Here's how the part is built. I have some questions about the finished solid (model axes, mm). Face numbers are marked on the shaded views. A direction names the side the tool comes from. Coordinates: 2 decimals unless noted, no trailing zeros. Write each loop counter-clockwise with the first axis right and the second up, starting at its lowest first coordinate (ties: lowest second). Pieces come first, ordered by that corner, then holes.
```python
from build123d import *

# Parameters (mm, degrees)
SKETCH1_W                               = 125
SKETCH1_H                               = 40
BOSS_EXTRUDE1_DEPTH                     = 10
BOSS_EXTRUDE2_DEPTH                     = 10
SKETCH9_W                               = 58.70504164
SKETCH9_H                               = 3.000259145
CUT_EXTRUDE1_DEPTH                      = 67
FILLET1_R                               = 3
FILLET2_R                               = 3
CBORE_FOR_M8_HEX_HEAD_BOLT1_D           = 9
CBORE_FOR_M8_HEX_HEAD_BOLT1_CBORE_D     = 18.01
CBORE_FOR_M8_HEX_HEAD_BOLT1_CBORE_DEPTH = 5.68


with BuildPart() as part:
    # Sketch1 → Boss-Extrude1 (new body)
    with BuildSketch(Plane(origin=(0, 0, 0), x_dir=(1, 0, 0), z_dir=(0, 1, 0))):
        with Locations((62.5, 20)):
            Rectangle(SKETCH1_W, SKETCH1_H)
    extrude(amount=BOSS_EXTRUDE1_DEPTH)

    # Sketch4 → Boss-Extrude2 (add)
    with BuildSketch(Plane.XY):
        with BuildLine():
            Line((30.012948081, 0), (69.987051919, 0))
            Line((69.987051919, 0), (69.987051919, 35))
            ThreePointArc((69.987051919, 35), (50, 54.987051919), (30.012948081, 35))
            Line((30.012948081, 35), (30.012948081, 0))
        make_face()
    extrude(amount=-BOSS_EXTRUDE2_DEPTH)

    # Sketch9 → Cut-Extrude1 (cut)
    with BuildSketch(Plane.XY):
        with Locations((53.635144719, 1.500129573)):
            Rectangle(SKETCH9_W, SKETCH9_H)
    extrude(amount=-CUT_EXTRUDE1_DEPTH, mode=Mode.SUBTRACT)

    # Fillet1
    fillet1_edges = [part.edges().sort_by_distance(p)[0] for p in [
        (0, 5, 0),
        (125, 5, 0),
        (125, 5, -40),
        (0, 5, -40),
    ]]
    fillet(fillet1_edges, radius=FILLET1_R)

    # Fillet2
    fillet2_edges = [part.edges().sort_by_distance(p)[0] for p in [
        (82.987665539, 0, -20),
        (24.282623899, 0, -20),
    ]]
    fillet(fillet2_edges, radius=FILLET2_R)

    # CBORE for M8 Hex Head Bolt1 (through all)
    with Locations(Plane(origin=(50, 35, -10), x_dir=(-1, 0, 0), z_dir=(0, 0, -1))):
        with Locations((0, 0)):
            CounterBoreHole(CBORE_FOR_M8_HEX_HEAD_BOLT1_D / 2, CBORE_FOR_M8_HEX_HEAD_BOLT1_CBORE_D / 2, CBORE_FOR_M8_HEX_HEAD_BOLT1_CBORE_DEPTH)


solid = part.part
```
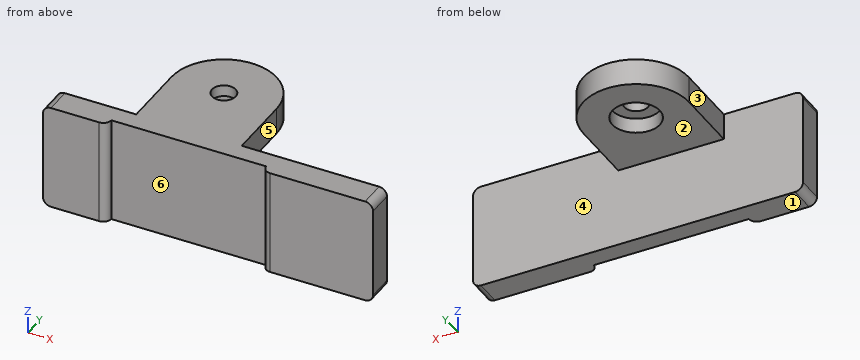
1) I need wall thicknesses on probe 1 along Y at (x, z) = (50, -6) (3 decimals); probe 2 along Y at (x, z) = (50, -1.75); probe 3 along Z at (x, y) = (51, 27). Which ranges of each line are inside material? Lowest first, please.
Values follow:
probe 1: y = 3 to 25.995, 44.005 to 54.987
probe 2: y = 3 to 30.5, 39.5 to 54.99
probe 3: z = -4.32 to 0
2) We'd pull the mould along X, two halves only. Please class the marked faces 4, 5 and 6: pulls with the +X half, pulls with the -X half, needs draft (parallel to the pull), parting line crosses it, or undercut.
Values follow:
face 4: needs draft
face 5: pulls with the +X half
face 6: undercut
3) Imagine slicing it at C-C on y = 23.5. Please give me the cut outline in (x, z), then the cut area to 3 significant figures.
Values follow:
outline: (30.01, -10) - (69.99, -10) - (69.99, 0) - (30.01, 0) - close
area: 400 mm2
4) Imagine slicing it at A-A on x = 50. Please give me the cut outline in (y, z) (3 decimals).
Values follow:
outline: (3, -40) - (10, -40) - (10, -10) - (25.995, -10) - (25.995, -4.32) - (30.5, -4.32) - (30.5, 0) - (3, 0) - close; (39.5, -4.32) - (44.005, -4.32) - (44.005, -10) - (54.987, -10) - (54.987, 0) - (39.5, 0) - close
5) On a 3-axis mill with a long thin cutter (end or side, diameter ignored), from which of +Z, -Z, +X, -X, +Y, -Y can I reach the whole of each face in a straight line? I mean the marked faces 1, 2 and 3. Say none if no direction works.
Values follow:
face 1: -Z, +X, -X, +Y, -Y
face 2: -Z, +X, -X, +Y
face 3: +Z, -Z, -X, +Y
6) Will these pins go through, and if not, where does the flat tip stop? pin 1 (20 mm diameter, centred on x = 51.5, z = -24.5, fed in from -Y); pin 2 (1 mm diameter, centred on x = 107, z = -24, fed in from +Y); pin 3 (12 mm diameter, centred on x = 46, y = 35.5, fed in from -Z).
Values follow:
pin 1: stops at y = 3
pin 2: stops at y = 10
pin 3: stops at z = -10
